```python
from build123d import *

# Parameters (mm, degrees)
F1_DEPTH = 1000
F2_R     = 3.25
F3_DEPTH = 25


with BuildPart() as f1:
    # F0 (on Right) → F1 (new body)
    with BuildSketch(Plane.YZ):
        Polygon((0, 62), (0, 0), (62, 0), (62, 20), (60, 20), (60, 2), (2, 2), (2, 62), align=None)
    extrude(amount=F1_DEPTH)

    # F2 (on face) → F3 (cut)
    with BuildSketch(Plane(origin=(0, 2, 0), x_dir=(-1, 0, 0), z_dir=(0, 1, 0))):
        with Locations((-980, 47)):
            Circle(F2_R)
        with Locations((-950, 47)):
            Circle(F2_R)
        with Locations((-980, 17)):
            Circle(F2_R)
        with Locations((-950, 17)):
            Circle(F2_R)
        with Locations((-50, 47)):
            Circle(F2_R)
        with Locations((-20, 47)):
            Circle(F2_R)
        with Locations((-20, 17)):
            Circle(F2_R)
        with Locations((-50, 17)):
            Circle(F2_R)
    extrude(amount=-F3_DEPTH, mode=Mode.SUBTRACT)


solid = f1.part
```
Design review of the part built by this model. Coordinates are the model's own, in mm. A direction names the side the tool comes from. Coordinates: 2 decimals unless noted, no trailing zeros. Write each loop counter-clockwise with the first axis right and the second up, starting at its lowest first coordinate (ties: lowest second). Pieces come first, ordered by that corner, then holes.
1) To check wall thickness, follow L1, parallel to Z at x = 20, y = 1.6; L2, parallel to Y at x = 608.5, z = 12; L3, parallel to Z at x = 333, y = 4.5. State the ranges of each line that lie inside material, in increasing order.
2) Insertion check: pin 1 (2 mm diameter, centred on x = 678, z = 32, fed in from +Y); pin 2 (1.6 mm diameter, centred on x = 330, y = 61.5, fed in from +Z); pin 3 (6 mm diameter, centred on x = 888, y = 42, fed in from +Z). Each pin has a flat end and moves straight along its axis. Give the tip position at first contact, or say it passes through.
3) Add section B-B (y = 36.5). Write out the cut boundary in (x, z).
4) Add section A-A (x = 326.5). Write out the cut boundary in (y, z).
5) Machinability: for faces 1 (the flat face through (493, 60, 11)), 2 (the flat face through (0, 22, 1)), which of the approach directions +Z, -Z, +X, -X, +Y, -Y give a long, thin tool a straight path to every point of the face, cutting with its end or side? Answer none if there is none.
6) Mouldability with a two-part tool opening along Y and no side actions: class faces 3 (the flat face through (493, 0, 31)), 4 (the flat face through (493, 2, 32)), 5 (the flat face through (493, 31, 0)) as +Y half, -Y half, draft (parallel to the pull), parting line (faces both ways), or undercut.
Check result:
1. L1: z = 0 to 13.75, 20.25 to 43.75, 50.25 to 62
1. L2: y = 0 to 2, 60 to 62
1. L3: z = 0 to 2
2. pin 1: stops at y = 2
2. pin 2: stops at z = 20
2. pin 3: stops at z = 2
3. outline: (0, 0) - (1000, 0) - (1000, 2) - (0, 2) - close
4. outline: (0, 0) - (62, 0) - (62, 20) - (60, 20) - (60, 2) - (2, 2) - (2, 62) - (0, 62) - close
5. face 1: +Z, +X, -X
5. face 2: +Z, -Z, -X, +Y, -Y
6. face 3: -Y half
6. face 4: undercut
6. face 5: draft
